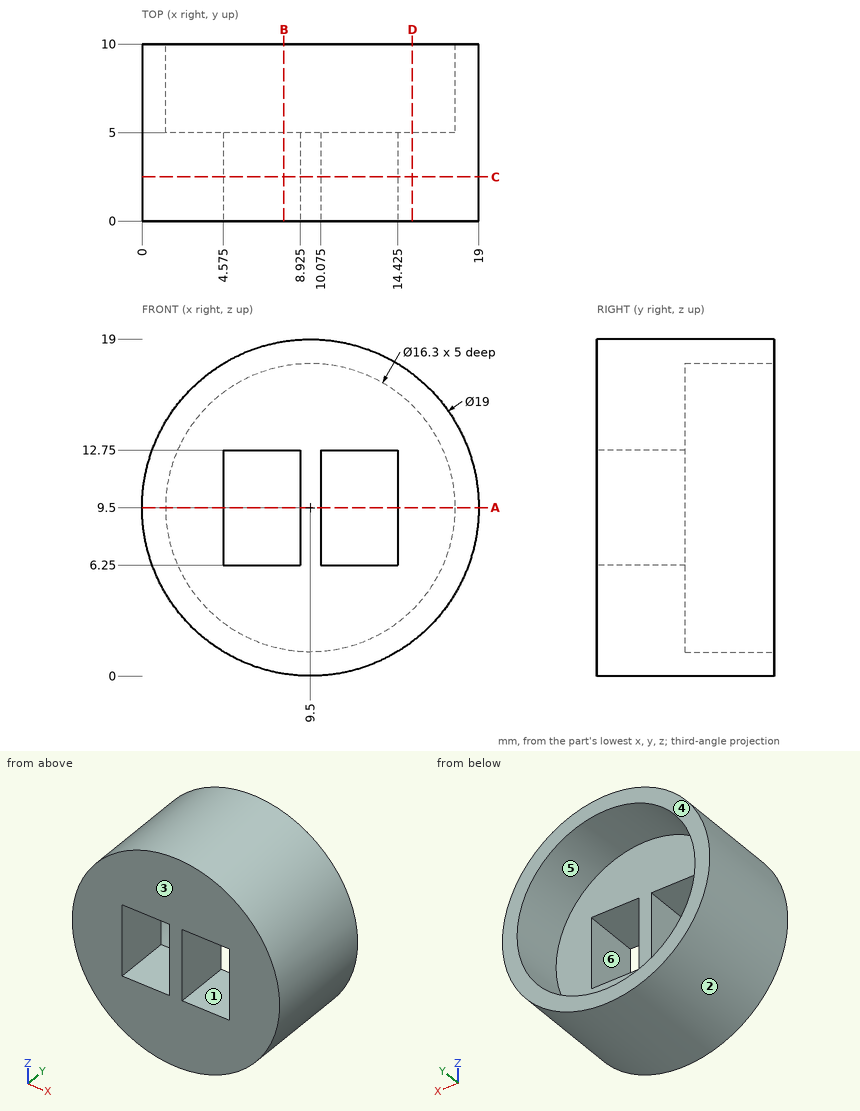
Answer from the drawing. Dimensions are ordinates in mm from the lowest x, y and z of the part. A direction names the side the tool comes from. Coordinates: 2 decimals unless noted, no trailing zeros. Loops run counter-clockwise (first coordinate to the right, second up) from the corner with the lowest first, then second, coordinate; pieces in that order, holes last. Notation, with made-up numbers: (-32.75, -4) -> (12.25, -4) arc R7 ccw to (12.25, 7) -> close; hole circle Ø6 at (-23.75, 12). An arc over 180 degrees is marked (long way). Return JSON: item names as keys, results as strings.
Item 1: For a pull along Z with two mould halves and no side action, classify the marked faces 1, 2 and 3 as +Z half, -Z half, draft (parallel to the pull), parting line (faces both ways), or undercut.
Answers:
{"face 1": "undercut", "face 2": "parting line", "face 3": "draft"}
Item 2: Find section C-C (y = 2.5). Determine the outline of the cut face in (x, z) (3 decimals), plus the area to 3 significant figures.
Answers:
{"outline": "circle Ø19 at (9.5, 9.5); hole (4.575, 6.25) -> (8.925, 6.25) -> (8.925, 12.75) -> (4.575, 12.75) -> close; hole (10.075, 6.25) -> (14.425, 6.25) -> (14.425, 12.75) -> (10.075, 12.75) -> close", "area": "227 mm2"}
Item 3: Find section D-D (x = 15.25). Determine the outline of the cut face in (y, z), plus the area to 3 significant figures.
Answers:
{"outline": "(0, 1.94) -> (10, 1.94) -> (10, 3.72) -> (5, 3.72) -> (5, 15.28) -> (10, 15.28) -> (10, 17.06) -> (0, 17.06) -> close", "area": "93.5 mm2"}
Item 4: Find the intervals of material crossed by probe 1 along Z at (x, y) = (9.5, 8.2); probe 2 along X at (y, z) = (2.75, 10.75) (3 decimals), in increasing order.
Answers:
{"probe 1": "z = 0 to 1.35, 17.65 to 19", "probe 2": "x = 0.083 to 4.575, 8.925 to 10.075, 14.425 to 18.917"}
Item 5: For the marked faces 4, 5 and 6, determine the directions among +Z, -Z, +X, -X, +Y, -Y from which every point of the face is accessible in a straight line to the end or side of a thin tool.
Answers:
{"face 4": "+Z, -Z, +X, -X, +Y", "face 5": "+Y", "face 6": "+Y, -Y"}
Item 6: Find section A-A (z = 9.5). Determine the outline of the cut face in (x, y) (3 decimals), plus the area to 3 significant figures.
Answers:
{"outline": "(0, 0) -> (4.575, 0) -> (4.575, 5) -> (1.35, 5) -> (1.35, 10) -> (0, 10) -> close; (8.925, 0) -> (10.075, 0) -> (10.075, 5) -> (8.925, 5) -> close; (14.425, 0) -> (19, 0) -> (19, 10) -> (17.65, 10) -> (17.65, 5) -> (14.425, 5) -> close", "area": "65.0 mm2"}
Item 7: Find section B-B (x = 8). Determine the outline of the cut face in (y, z).
Answers:
{"outline": "(0, 0.12) -> (10, 0.12) -> (10, 1.49) -> (5, 1.49) -> (5, 6.25) -> (0, 6.25) -> close; (0, 12.75) -> (5, 12.75) -> (5, 17.51) -> (10, 17.51) -> (10, 18.88) -> (0, 18.88) -> close"}
Item 8: Flat-ended cylindrical pins translate along their axes: P1, Ø1.5, axis at y = 2.5, z = 10.5, coming from the +X side; P2, Ø1.3, axis at x = 8, y = 2, coming from the -Z side; P3, Ø5, axis at y = 6.5, z = 16, coming from the -X side; P4, Ø4, axis at y = 3.5, z = 8.5, coming from the -X side. Find the tip coordinate at first contact, or state that the pin passes through.
Answers:
{"P1": "stops at x = 19", "P2": "stops at z = 0.04", "P3": "stops at x = 0.88", "P4": "stops at x = 0"}
